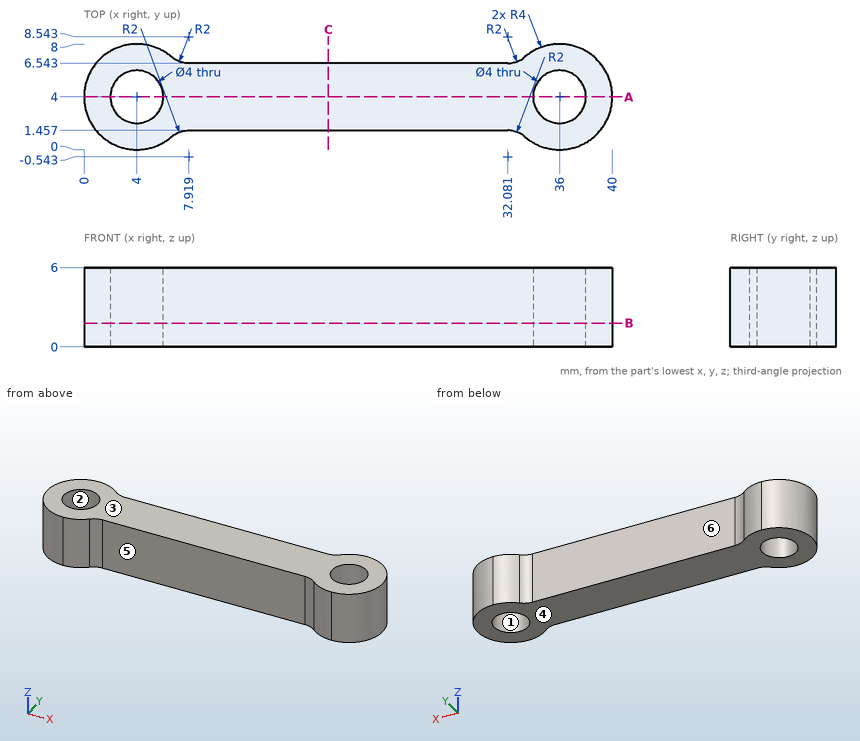
The drawing under review shows one solid part. Ordinate dimensions are in mm from its lowest x, y, z. A direction names the side the tool comes from. Round coordinates to 2 decimals unless told otherwise and drop trailing zeros. Loops run counter-clockwise (first coordinate to the right, second up) from the corner with the lowest first, then second, coordinate; pieces in that order, holes last. Notation, with made-up numbers: M 40.5,-27.75 L 97.5,-27.75 A18 ccw 97.5,7.25 Z; hole C 59.25,12.5 d1. An arc over 180 degrees is marked long. Answer as CSV lines item,"result". Start each with the question number.
Item 1: Consider section B-B (z = 1.8). Write out the cut boundary in (x, y).
Item 2: Consider section A-A (y = 4). Write out the cut boundary in (x, z), then the cut area to 3 significant figures.
Item 3: Insertion check: P1, Ø2.5, axis at x = 36, y = 4, coming from the -Z side; P2, Ø1.8, axis at x = 21.5, z = 1.5, coming from the -Y side; P3, Ø2, axis at x = 17.5, z = 3, coming from the +Y side; P4, Ø2, axis at y = 1.5, z = 4.5, coming from the -X side. Each pin has a flat end and moves straight along its axis. Give the tip position at first contact, or say it passes through.
Item 4: Consider section C-C (x = 18.5). Write out the cut boundary in (y, z).
Item 5: Mouldability with a two-part tool opening along X and no side actions: class the marked faces 1, 2 and 3 as released by +X, released by -X, zero draft, split by the parting line, or undercut.
Item 6: Wall thickness on line 1 (Y direction, x = 36, z = 2.7); line 2 (X direction, y = 3.5, z = 0.45); line 3 (X direction, y = 5, z = 3.55): over which ranges is each line inside the solid? List them lowest first. Write a range as [from, to].
Item 7: For the marked faces 4, 5 and 6, list the 3-axis set-ups (+Z, -Z, +X, -X, +Y, -Y) from which the entire face can be reached by the end or side of a thin tool; tool diameter is ignored.
Answer:
1,outline,"M 6.61,0.97 A2 cw 7.92,1.46 L 32.08,1.46 A2 cw 33.39,0.97 A4 ccw long 33.39,7.03 A2 cw 32.08,6.54 L 7.92,6.54 A2 cw 6.61,7.03 A4 ccw long Z; hole C 4,4 d4; hole C 36,4 d4"
2,outline,"M 0,0 L 2,0 L 2,6 L 0,6 Z; M 6,0 L 34,0 L 34,6 L 6,6 Z; M 38,0 L 40,0 L 40,6 L 38,6 Z"
2,area,"192 mm^2"
3,P1,"passes through"
3,P2,"stops at y = 1.46"
3,P3,"stops at y = 6.54"
3,P4,"stops at x = 0.29"
4,outline,"M 1.46,0 L 6.54,0 L 6.54,6 L 1.46,6 Z"
5,face 1,"undercut"
5,face 2,"undercut"
5,face 3,"zero draft"
6,line 1,"y = [0, 2], [6, 8]"
6,line 2,"x = [0.03, 2.06], [5.94, 34.06], [37.94, 39.97]"
6,line 3,"x = [0.13, 2.27], [5.73, 34.27], [37.73, 39.87]"
7,face 4,"-Z, +X, -X, +Y, -Y"
7,face 5,"+Z, -Z, -Y"
7,face 6,"+Z, -Z, +Y"
